For this review, take the finished solid that the model builds, in its own axes (mm). Face numbers are marked on the shaded views. Give positions to 0.01 mm unless a question says otherwise; leave off trailing zeros. Order: outer loops, then holes, each group sorted by start corner. A loop starts at its lowest first (then second) coordinate and runs counter-clockwise, first axis right, second up. Notation, with made-up numbers: (0.5, 30) - (10.5, 30) arc R18 cw to (10.5, 38) - close; hole circle Ø10 at (-40, 8). An arc over 180 degrees is marked (long way). Use a Markdown table: item, result. Add a question column.
1) We need section C-C on x = 94. Write out the cut boundary in (y, z).
2) We need section A-A on y = 0. Write out the cut boundary in (x, z), then the cut area to 3 significant figures.
3) Wall thickness on L1, parallel to Y at x = 94, z = 0; L2, parallel to Y at x = 32, z = 0; L3, parallel to X at y = 11, z = 4: over which ranges is each line inside the solid? List them lowest first.
4) Mouldability with a two-part tool opening along Y and no side actions: class the marked faces 1, 2 and 3 as released by +Y, released by -Y, zero draft, split by the parting line, or undercut.
5) Clearance check with flat-ended pins moving along their axes: P1, Ø19, axis at y = 0, z = 0, coming from the -X side; P2, Ø1, axis at x = 94, y = -15, coming from the -Z side (3 decimals); P3, Ø10, axis at x = 27.5, z = 21, coming from the +Y side. State where each tip first meets the part, or that it passes through.
```python
from build123d import *


with BuildPart() as part:
    # 草图1 → 旋转1 (revolve)
    with BuildSketch(Plane.XY, mode=Mode.PRIVATE) as revolve_1_sk:
        with BuildLine():
            Line((0, 13), (0, 24))
            ThreePointArc((0, 24), (4, 28), (8, 24))
            Line((8, 24), (8, 22))
            ThreePointArc((8, 22), (8.585786438, 20.585786438), (10, 20))
            Line((10, 20), (116, 20))
            ThreePointArc((116, 20), (118.828427125, 18.828427125), (120, 16))
            Line((120, 16), (120, 2))
            Line((120, 2), (117, 2))
            Line((117, 2), (60, 2))
            Line((60, 2), (60, 12))
            Line((60, 12), (1, 12))
            Line((1, 12), (0, 13))
        make_face()
    revolve(revolve_1_sk.sketch.rotate(Axis((0, 0, 0), (1, 0, 0)), 90), axis=Axis((0, 0, 0), (1, 0, 0)))


solid = part.part
```
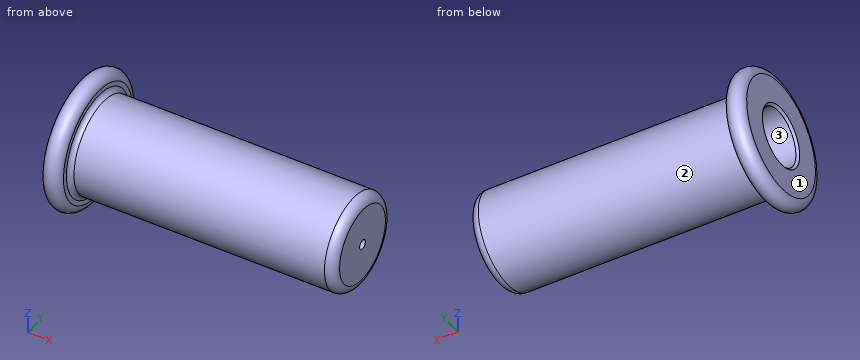
Checked values:
| question | item | result |
|---|---|---|
| 1 | outline | circle Ø40 at (0, 0); hole circle Ø4 at (0, 0) |
| 2 | outline | (0, -24) arc R4 ccw to (8, -24) - (8, -22) arc R2 cw to (10, -20) - (116, -20) arc R4 ccw to (120, -16) - (120, -2) - (60, -2) - (60, -12) - (1, -12) - (0, -13) - close; (0, 13) - (1, 12) - (60, 12) - (60, 2) - (120, 2) - (120, 16) arc R4 ccw to (116, 20) - (10, 20) arc R2 cw to (8, 22) - (8, 24) arc R4 ccw to (0, 24) - close |
| 2 | area | 3,230 mm² |
| 3 | L1 | -20 to -2, 2 to 20 |
| 3 | L2 | -20 to -12, 12 to 20 |
| 3 | L3 | 60 to 120 |
| 4 | face 1 | zero draft |
| 4 | face 2 | split by the parting line |
| 4 | face 3 | undercut |
| 5 | P1 | x = 60 |
| 5 | P2 | z = -13.775 |
| 5 | P3 | y = 12 |
